```python
from build123d import *

# Parameters (mm, degrees)
F0_W          = 13.97
F0_H          = 5.08
F1_DEPTH      = 6
F3_DEPTH      = 5.08
F4_R          = 3.175
F5_DEPTH      = 11.43
F6_R          = 1.27
F7_DEPTH      = 7.874
F8_R          = 2.54
F9_R          = 0.254
F10_T2_ANGLE  = 160.8118635463
F10_T6_ANGLE  = 359.64
F10_T11_ANGLE = 359.64


# Not quite as in the source:
# - a fillet or chamfer that OpenCascade refuses, or shapes differently, is made with other operations: its cross-section is extruded or revolved along the edge and cut away or added


with BuildPart() as f1:
    # F0 (on Top) → F1 (new body)
    with BuildSketch(Plane.XY):
        with Locations((-6.985, -2.54)):
            Rectangle(F0_W, F0_H)
    extrude(amount=F1_DEPTH)

    # F2 (on face) → F3 (join)
    with BuildSketch(Plane.XZ.offset(5.08)):
        Polygon((-11.43, 6), (-13.97, 6), (-13.97, 0), (-11.43, 0), (-11.43, 1.7556592107), align=None)
    extrude(amount=F3_DEPTH)

    # F4 (on face) → F5 (cut)
    with BuildSketch(Plane.YZ):
        with Locations((-5.08, 3)):
            Circle(F4_R)
    extrude(amount=-F5_DEPTH, mode=Mode.SUBTRACT)

    # F6 (on face) → F7 (cut)
    with BuildSketch(Plane.XZ.offset(10.16)):
        with Locations((-11.43, 3)):
            Circle(F6_R)
    extrude(amount=-F7_DEPTH, mode=Mode.SUBTRACT)

    # F8
    f8_edges = [f1.edges().sort_by_distance(p)[0] for p in [
        (-6.985, 0, 6),
        (-6.985, 0, 0),
    ]]
    fillet(f8_edges, radius=F8_R)

    # F9
    f9_edges = [f1.edges().sort_by_distance(p)[0] for p in [
        (-11.43, -10.16, 5.135),
        (-12.7, -10.16, 6),
        (-12.7, -10.16, 3),
        (-11.43, -10.16, 0.865),
        (-12.7, -10.16, 0),
        (-13.97, -10.16, 3),
        (-13.97, -6.35, 6),
        (-11.43, -7.100234, 6),
        (-11.43, -7.100234, 0),
        (-11.43, -6.223, 1.73),
        (-11.43, -6.223, 4.27),
        (-5.715, -4.040469, 6),
        (-5.715, -4.040469, 0),
        (-13.97, -6.35, 0),
        (-13.97, -0.743949, 0.743949),
        (-13.97, 0, 3),
        (-13.97, -0.743949, 5.256051),
    ]]
    fillet(f9_edges, radius=F9_R)

    # F10: fillet of radius 0.508 on 1 edges, made by hand

    # F10_s1 → F10_t2 (revolve)
    with BuildSketch(Plane(origin=(-10.6194933514, 0, -1.7950219978), x_dir=(0, 1, 0), z_dir=(0.9860132972, 0, 0.1666666667))):
        with BuildLine():
            ThreePointArc((-2.286, 5.6250398915), (-2.4347897552, 5.9842501364), (-2.794, 6.1330398915))
            Line((-2.794, 6.1330398915), (-2.286, 6.1330398915))
            Line((-2.286, 6.1330398915), (-2.286, 5.6250398915))
        make_face()
    revolve(axis=Axis((-11.43, -2.286, 3), (0, -1, 0)), revolution_arc=F10_T2_ANGLE)


with BuildPart() as f10_tool4:
    # F10_s5 → F10_t6 (revolve)
    with BuildSketch(Plane(origin=(-10.6699629137, 0, -1.7346683419), x_dir=(0, 1, 0), z_dir=(0.9870410248, 0, 0.1604681133))):
        with BuildLine():
            ThreePointArc((-2.794, 6.065243527), (-2.4347897552, 5.9164537719), (-2.286, 5.557243527))
            Line((-2.286, 5.557243527), (-2.286, 6.065243527))
            Line((-2.286, 6.065243527), (-2.794, 6.065243527))
        make_face()
    revolve(axis=Axis((-11.684, -2.286, 4.5026842649), (0, 1, 0)), revolution_arc=F10_T6_ANGLE)

    split(bisect_by=Plane.YZ.offset(-11.43), keep=Keep.BOTTOM)


with BuildPart() as f1_1:
    add(f1.part)

    # F10_t3: union F10_tool4
    add(f10_tool4.part)


with BuildPart() as f10_tool9:
    # F10_s10 → F10_t11 (revolve)
    with BuildSketch(Plane(origin=(-11.6202945797, 0, 1.8891684342), x_dir=(0, 1, 0), z_dir=(0.9870410248, 0, -0.1604681133))):
        with BuildLine():
            ThreePointArc((-2.794, -0.1429973783), (-2.4347897552, 0.0057923768), (-2.286, 0.3650026217))
            Line((-2.286, 0.3650026217), (-2.286, -0.1429973783))
            Line((-2.286, -0.1429973783), (-2.794, -0.1429973783))
        make_face()
    revolve(axis=Axis((-11.684, -2.286, 1.4973157351), (0, -1, 0)), revolution_arc=F10_T11_ANGLE)

    split(bisect_by=Plane.YZ.offset(-11.43), keep=Keep.BOTTOM)


with BuildPart() as f1_2:
    add(f1_1.part)

    # F10_t8: union F10_tool9
    add(f10_tool9.part)


solid = f1_2.part
```
The listing builds one solid part. Answer for the finished solid, in the listing's coordinates (mm). A direction names the side the tool comes from. Round coordinates to 2 decimals unless told otherwise and drop trailing zeros. Loops run counter-clockwise (first coordinate to the right, second up) from the corner with the lowest first, then second, coordinate; pieces in that order, holes last. Notation, with made-up numbers: (3.5, 70) - (18.5, 70) arc R14 cw to (18.5, 94) - close; hole circle Ø8 at (-29.75, 67.25). An arc over 180 degrees is marked (long way). Return JSON: item names as keys, results as strings. Group by question number.
1. Each of these flat-tipped pins is pushed along its axis until it touches: P1, Ø1, axis at x = -10.5, z = 5, coming from the -Y side; P2, Ø0.6, axis at x = -12, z = 2.5, coming from the -Y side. Where does it stop, or does it pass through?
2. The part is cut by section A-A on y = -5.25. Determine the outline of the cut face in (x, z).
3. Which of the six approach directions +Z, -Z, +X, -X, +Y, -Y give full straight-line access (tool end or side, diameter ignored) to faces 1 (the flat face through (-7, 0, 3)), 2 (the cylindrical face through (-12.7, -6.4, 3))?
4. The part is cut by section B-B on x = -9. Determine the outline of the cut face in (y, z) (3 decimals).
5. The mould has two halves that part along Z. Classify faces 3 (the cylindrical face through (-6.762, -0.724, 0.764)), 4 (the flat face through (0, -1, 3)), 5 (the cylindrical face through (-5.635, -1.905, 2.959)), 6 (the cylindrical face through (-6.762, -0.764, 5.276)): pulls with the +Z half, pulls with the -Z half, needs draft (parallel to the pull), parting line crosses it, or undercut.
6. Consider probe 1 along Y at (x, z) = (-1.25, 2.9); probe 2 along Z at (x, y) = (-10, -2.5); probe 3 along X at (y, z) = (-5.75, 5.2). Determine where each line is inside the solid, lowest interval first.
Resolved:
{
 "1": {"P1": "stops at y = -3.12", "P2": "stops at y = -2.38"},
 "2": {"outline": "(-13.97, 0.25) arc R0.25 ccw to (-13.72, 0) - (-11.68, 0) arc R0.25 ccw to (-11.43, 0.25) - (-11.43, 1.5) arc R0.25 ccw to (-11.64, 1.75) arc R1.27 cw to (-11.64, 4.25) arc R0.25 ccw to (-11.43, 4.5) - (-11.43, 5.75) arc R0.25 ccw to (-11.68, 6) - (-13.72, 6) arc R0.25 ccw to (-13.97, 5.75) - close"},
 "3": {"face 1": "+Z, -Z, +X, -X, +Y", "face 2": "+X, -Y"},
 "4": {"outline": "(-3.178, 0.457) arc R0.254 ccw to (-3.026, 0) - (-2.54, 0) arc R2.54 ccw to (0, 2.54) - (0, 3.46) arc R2.54 ccw to (-2.54, 6) - (-3.026, 6) arc R0.254 ccw to (-3.178, 5.543) arc R3.175 cw to start"},
 "5": {"face 3": "pulls with the -Z half", "face 4": "needs draft", "face 5": "undercut", "face 6": "pulls with the +Z half"},
 "6": {"probe 1": "y = -1.91 to 0", "probe 2": "z = 0 to 1.15, 4.85 to 6", "probe 3": "x = -13.97 to -11.43"}
}
